Read the model definition and answer for the solid it produces. Units are mm, in the model's axes. Coordinates: 2 decimals unless noted, no trailing zeros. Order: outer loops, then holes, each group sorted by start corner. A loop starts at its lowest first (then second) coordinate and runs counter-clockwise, first axis right, second up. Notation, with made-up numbers: (-21, 47) - (-17, 47) arc R13 ccw to (-17, 56) - close; hole circle Ø11 at (-20.5, 44). An arc over 180 degrees is marked (long way). Use one line per item in the form item = value.
```python
from build123d import *

# Parameters (mm, degrees)
SKETCH1_W           = 75.25
SKETCH1_H           = 191
SKETCH1_R           = 5.75
BOSS_EXTRUDE1_DEPTH = 15


with BuildPart() as part:
    # Sketch1 → Boss-Extrude1 (new body)
    with BuildSketch(Plane(origin=(0, 0, 0), x_dir=(1, 0, 0), z_dir=(0, 1, 0))):
        Rectangle(SKETCH1_W, SKETCH1_H)
        with Locations(Location((-26.025, 85.5, 0), (0, 0, 270))):
            Circle(SKETCH1_R, mode=Mode.SUBTRACT)
        with Locations(Location((-8.675, 85.5, 0), (0, 0, 270))):
            Circle(SKETCH1_R, mode=Mode.SUBTRACT)
        with Locations(Location((8.675, 85.5, 0), (0, 0, 270))):
            Circle(SKETCH1_R, mode=Mode.SUBTRACT)
        with Locations(Location((26.025, 85.5, 0), (0, 0, 270))):
            Circle(SKETCH1_R, mode=Mode.SUBTRACT)
        with Locations(Location((-26.025, 70.5, 0), (0, 0, 270))):
            Circle(SKETCH1_R, mode=Mode.SUBTRACT)
        with Locations(Location((-8.675, 70.5, 0), (0, 0, 270))):
            Circle(SKETCH1_R, mode=Mode.SUBTRACT)
        with Locations(Location((8.675, 70.5, 0), (0, 0, 270))):
            Circle(SKETCH1_R, mode=Mode.SUBTRACT)
        with Locations(Location((26.025, 70.5, 0), (0, 0, 270))):
            Circle(SKETCH1_R, mode=Mode.SUBTRACT)
        with Locations(Location((-26.025, 55.5, 0), (0, 0, 270))):
            Circle(SKETCH1_R, mode=Mode.SUBTRACT)
        with Locations(Location((-8.675, 55.5, 0), (0, 0, 270))):
            Circle(SKETCH1_R, mode=Mode.SUBTRACT)
        with Locations(Location((8.675, 55.5, 0), (0, 0, 270))):
            Circle(SKETCH1_R, mode=Mode.SUBTRACT)
        with Locations(Location((26.025, 55.5, 0), (0, 0, 270))):
            Circle(SKETCH1_R, mode=Mode.SUBTRACT)
        with Locations(Location((-26.025, 40.5, 0), (0, 0, 270))):
            Circle(SKETCH1_R, mode=Mode.SUBTRACT)
        with Locations(Location((-8.675, 40.5, 0), (0, 0, 270))):
            Circle(SKETCH1_R, mode=Mode.SUBTRACT)
        with Locations(Location((8.675, 40.5, 0), (0, 0, 270))):
            Circle(SKETCH1_R, mode=Mode.SUBTRACT)
        with Locations(Location((26.025, 40.5, 0), (0, 0, 270))):
            Circle(SKETCH1_R, mode=Mode.SUBTRACT)
        with Locations(Location((-26.025, 25.5, 0), (0, 0, 270))):
            Circle(SKETCH1_R, mode=Mode.SUBTRACT)
        with Locations(Location((-8.675, 25.5, 0), (0, 0, 270))):
            Circle(SKETCH1_R, mode=Mode.SUBTRACT)
        with Locations(Location((8.675, 25.5, 0), (0, 0, 270))):
            Circle(SKETCH1_R, mode=Mode.SUBTRACT)
        with Locations(Location((26.025, 25.5, 0), (0, 0, 270))):
            Circle(SKETCH1_R, mode=Mode.SUBTRACT)
        with Locations(Location((-26.025, 10.5, 0), (0, 0, 270))):
            Circle(SKETCH1_R, mode=Mode.SUBTRACT)
        with Locations(Location((-8.675, 10.5, 0), (0, 0, 270))):
            Circle(SKETCH1_R, mode=Mode.SUBTRACT)
        with Locations(Location((8.675, 10.5, 0), (0, 0, 270))):
            Circle(SKETCH1_R, mode=Mode.SUBTRACT)
        with Locations(Location((26.025, 10.5, 0), (0, 0, 270))):
            Circle(SKETCH1_R, mode=Mode.SUBTRACT)
        with Locations(Location((-26.025, -4.5, 0), (0, 0, 270))):
            Circle(SKETCH1_R, mode=Mode.SUBTRACT)
        with Locations(Location((-8.675, -4.5, 0), (0, 0, 270))):
            Circle(SKETCH1_R, mode=Mode.SUBTRACT)
        with Locations(Location((8.675, -4.5, 0), (0, 0, 270))):
            Circle(SKETCH1_R, mode=Mode.SUBTRACT)
        with Locations(Location((26.025, -4.5, 0), (0, 0, 270))):
            Circle(SKETCH1_R, mode=Mode.SUBTRACT)
        with Locations(Location((-26.025, -19.5, 0), (0, 0, 270))):
            Circle(SKETCH1_R, mode=Mode.SUBTRACT)
        with Locations(Location((-8.675, -19.5, 0), (0, 0, 270))):
            Circle(SKETCH1_R, mode=Mode.SUBTRACT)
        with Locations(Location((8.675, -19.5, 0), (0, 0, 270))):
            Circle(SKETCH1_R, mode=Mode.SUBTRACT)
        with Locations(Location((26.025, -19.5, 0), (0, 0, 270))):
            Circle(SKETCH1_R, mode=Mode.SUBTRACT)
        with Locations(Location((-26.025, -34.5, 0), (0, 0, 270))):
            Circle(SKETCH1_R, mode=Mode.SUBTRACT)
        with Locations(Location((-8.675, -34.5, 0), (0, 0, 270))):
            Circle(SKETCH1_R, mode=Mode.SUBTRACT)
        with Locations(Location((8.675, -34.5, 0), (0, 0, 270))):
            Circle(SKETCH1_R, mode=Mode.SUBTRACT)
        with Locations(Location((26.025, -34.5, 0), (0, 0, 270))):
            Circle(SKETCH1_R, mode=Mode.SUBTRACT)
        with Locations(Location((-26.025, -49.5, 0), (0, 0, 270))):
            Circle(SKETCH1_R, mode=Mode.SUBTRACT)
        with Locations(Location((-8.675, -49.5, 0), (0, 0, 270))):
            Circle(SKETCH1_R, mode=Mode.SUBTRACT)
        with Locations(Location((8.675, -49.5, 0), (0, 0, 270))):
            Circle(SKETCH1_R, mode=Mode.SUBTRACT)
        with Locations(Location((26.025, -49.5, 0), (0, 0, 270))):
            Circle(SKETCH1_R, mode=Mode.SUBTRACT)
        with Locations(Location((-26.025, -64.5, 0), (0, 0, 270))):
            Circle(SKETCH1_R, mode=Mode.SUBTRACT)
        with Locations(Location((-8.675, -64.5, 0), (0, 0, 270))):
            Circle(SKETCH1_R, mode=Mode.SUBTRACT)
        with Locations(Location((8.675, -64.5, 0), (0, 0, 270))):
            Circle(SKETCH1_R, mode=Mode.SUBTRACT)
        with Locations(Location((26.025, -64.5, 0), (0, 0, 270))):
            Circle(SKETCH1_R, mode=Mode.SUBTRACT)
        with Locations(Location((-26.025, -79.5, 0), (0, 0, 270))):
            Circle(SKETCH1_R, mode=Mode.SUBTRACT)
        with Locations(Location((-8.675, -79.5, 0), (0, 0, 270))):
            Circle(SKETCH1_R, mode=Mode.SUBTRACT)
        with Locations(Location((8.675, -79.5, 0), (0, 0, 270))):
            Circle(SKETCH1_R, mode=Mode.SUBTRACT)
        with Locations(Location((26.025, -79.5, 0), (0, 0, 270))):
            Circle(SKETCH1_R, mode=Mode.SUBTRACT)
    extrude(amount=BOSS_EXTRUDE1_DEPTH)


solid = part.part
```
(1) Section C-C, the plane x = 11.5 is taken. State how many separate pieces and enclosed holes the cut face has, then the cut area to 3 significant figures.
Answer list:
separate_pieces = 13
enclosed_holes = 0
area = 1,060 mm2
(2) Section B-B, the plane z = 36 is taken. Write down the section's boundary in (x, y) (3 decimals), then the cut area to 3 significant figures.
Answer list:
outline = (-37.625, 0) - (-31.576, 0) - (-31.576, 15) - (-37.625, 15) - close; (-20.474, 0) - (-14.226, 0) - (-14.226, 15) - (-20.474, 15) - close; (-3.124, 0) - (3.124, 0) - (3.124, 15) - (-3.124, 15) - close; (14.226, 0) - (20.474, 0) - (20.474, 15) - (14.226, 15) - close; (31.576, 0) - (37.625, 0) - (37.625, 15) - (31.576, 15) - close
area = 463 mm2
(3) Given pin 1 Ø7 at (x, z) = (-8.675, -25.5) entering from -Y, flat-ended and moving along its own axis, determine where the tip first touches the part or whether it passes through.
Answer list:
pin_1 = through
(4) Straight lines are drawn through the part: L1, parallel to X at y = 2.5, z = -55 (3 decimals); L2, parallel to X at y = 5.5, z = -15 (3 decimals). For each, find the intervals that lie inside material, in ascending order.
Answer list:
L1 = -37.625 to -31.753, -20.297 to -14.403, -2.947 to 2.947, 14.403 to 20.297, 31.753 to 37.625
L2 = -37.625 to -29.604, -22.446 to -12.254, -5.096 to 5.096, 12.254 to 22.446, 29.604 to 37.625
(5) Section A-A, the plane z = -25.5 is taken. Write down the section's boundary in (x, y) (3 decimals).
Answer list:
outline = (-37.625, 0) - (-31.775, 0) - (-31.775, 15) - (-37.625, 15) - close; (-20.275, 0) - (-14.425, 0) - (-14.425, 15) - (-20.275, 15) - close; (-2.925, 0) - (2.925, 0) - (2.925, 15) - (-2.925, 15) - close; (14.425, 0) - (20.275, 0) - (20.275, 15) - (14.425, 15) - close; (31.775, 0) - (37.625, 0) - (37.625, 15) - (31.775, 15) - close
(6) The mould has two halves that part along Z. Classify faces 1 (the flat face through (37.625, 7, 1)), 2 (the flat face through (-1, 7, -95.5)), 3 (the cylindrical face through (-14.3, 7.4, 33.3)): +Z half, -Z half, draft (parallel to the pull), parting line (faces both ways), or undercut.
Answer list:
face_1 = draft
face_2 = -Z half
face_3 = undercut
